Geometry check sheet. Reference: the model listing, model coordinates, mm. A direction names the side the tool comes from. Coordinates: 2 decimals unless noted, no trailing zeros. Write each loop counter-clockwise with the first axis right and the second up, starting at its lowest first coordinate (ties: lowest second). Pieces come first, ordered by that corner, then holes.
Autodesk Inventor part; units mm, degrees
ref_plane "YZ Plane" through (0, 0, 0) normal (1, 0, 0) x (0, 1, 0)
ref_plane "XZ Plane" through (0, 0, 0) normal (0, 1, 0) x (-1, 0, 0)
ref_plane "XY Plane" through (0, 0, 0) normal (0, 0, 1) x (1, 0, 0)
sketch "Sketch5" plane through (0, 0, 0) normal (0, 0, 1) x (1, 0, 0)
  circle A0 centre (0, 0) radius 3.75
  dimension "d11" = 7.5
extrude "Extrusion4" add sketch "Sketch5" along normal blind 5
sketch "Sketch6" plane through (0, 0, 5) normal (0, 0, 1) x (1, 0, 0)
  line L0 (0, 0) -> (-10, 0)
  line L1 (-10, 0) -> (-10, 10)
  line L2 (-10, 10) -> (10, 10)
  line L3 (10, 10) -> (10, -10)
  line L4 (10, -10) -> (-10, -10)
  line L5 (-10, -10) -> (-10, 0)
  dimension "d19" = 10
  dimension "d20" = 10
  dimension "d21" = 20
  dimension "d22" = 20
  dimension "d23" = 20
extrude "Extrusion5" add sketch "Sketch6" along normal blind 20
fillet "Fillet1" radius 2 12 edges at (-10, 0, 5) (0, -10, 5) (-10, -10, 15) (0, 10, 5) (10, 10, 15) (10, 0, 5) (-10, 10, 15) (-10, 0, 25) (0, 10, 25) (10, 0, 25) (0, -10, 25) (10, -10, 15)
properties part number "Holder"
1. Sectioned sample at B-B, the plane y = 0. Record the boundary of the cut face in (x, z).
Computed values:
outline: (-10, 7) arc R2 ccw to (-8, 5) - (-3.75, 5) - (-3.75, 0) - (3.75, 0) - (3.75, 5) - (8, 5) arc R2 ccw to (10, 7) - (10, 23) arc R2 ccw to (8, 25) - (-8, 25) arc R2 ccw to (-10, 23) - close
2. Gauge pin test, flat end, axial feed: pin 1 Ø3 at (x, y) = (6.5, -7.5) entering from -Z. Record the tip position at first contact, or that the pin passes through.
Computed values:
pin 1: stops at z = 5
3. Thickness scan on line 1 along Z through (x, y) = (0.25, -5); line 2 along X through (y, z) = (-3.25, 2.75); line 3 along X through (y, z) = (-8.5, 24.25). Record the ranges inside material, lowest first.
Computed values:
line 1: z = 5 to 25
line 2: x = -1.87 to 1.87
line 3: x = -9.48 to 9.48
4. Sectioned sample at C-C, the plane z = 3. Record the boundary of the cut face in (x, y).
Computed values:
outline: circle Ø7.5 at (0, 0)
5. Sectioned sample at A-A, the plane x = 4.5. Record the boundary of the cut face in (y, z), and give its area (3 significant figures).
Computed values:
outline: (-10, 7) arc R2 ccw to (-8, 5) - (8, 5) arc R2 ccw to (10, 7) - (10, 23) arc R2 ccw to (8, 25) - (-8, 25) arc R2 ccw to (-10, 23) - close
area: 397 mm2
6. Access from +Z, -Z, +X, -X, +Y, -Y to the whole of each face (thin tool, end or side, straight path). Record for faces 1 (the cylindrical face through (-3.746, -0.165, 2.465)), 2 (the cylindrical face through (-0.11, -9.43, 24.4)).
Computed values:
face 1: -Z
face 2: +Z, +X, -X, -Y
